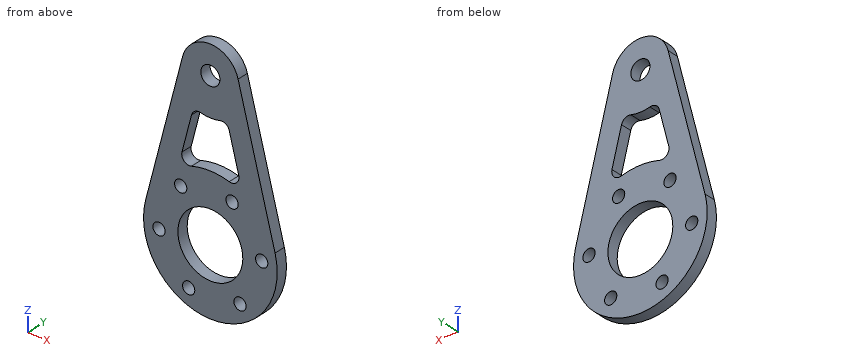
```python
from build123d import *

# Parameters (mm, degrees)
SKETCH_1_R               = 17.5
SKETCH_1_R_2             = 7.5
SKETCH_1_R_3             = 2.5
EXTRUDE_1_DEPTH          = 3
SKETCH_2_R               = 1.6
SKETCH_2_R_2             = 8.5
CUT_EXTRUDE_1_DEPTH      = 4
PATTERN_CIRCULAR_1_COUNT = 2
CUT_EXTRUDE_2_DEPTH      = 4
FILLET_1_R               = 2


with BuildPart() as part:
    # 草图1 → 凸台-拉伸1 (new body)
    # profile 1 of 3: a face of its own
    with BuildSketch(Plane(origin=(0, 0, 0), x_dir=(1, 0, 0), z_dir=(0, 1, 0))):
        Circle(SKETCH_1_R)
    # profile 2 of 3: a face of its own
    with BuildSketch(Plane(origin=(0, 0, 0), x_dir=(1, 0, 0), z_dir=(0, 1, 0))):
        with BuildLine():
            Line((-16.94430214, -4.375), (-7.261843774, -41.875))
            ThreePointArc((-7.261843774, -41.875), (-0.945032194, -32.559777278), (7.5, -40))
            ThreePointArc((7.5, -40), (7.440222722, -40.945032194), (7.261843774, -41.875))
            Line((7.261843774, -41.875), (16.94430214, -4.375))
            ThreePointArc((16.94430214, -4.375), (0, -17.5), (-16.94430214, -4.375))
        make_face()
    # profile 3 of 3: a face of its own
    with BuildSketch(Plane(origin=(0, 0, 0), x_dir=(1, 0, 0), z_dir=(0, 1, 0))):
        with Locations((0, -40)):
            Circle(SKETCH_1_R_2)
        with Locations(Location((0, -40, 0), (0, 0, 270))):
            Circle(SKETCH_1_R_3, mode=Mode.SUBTRACT)
    extrude(amount=EXTRUDE_1_DEPTH)

    # 草图2 → 切除-拉伸1 (cut)
    with BuildSketch(Plane.XZ):
        with Locations(Location((13.446267609, 1.203281922, 0), (0, 0, 270))):
            Circle(SKETCH_2_R)
        with Locations(Location((-5.681061093, -12.246450296, 0), (0, 0, 270))):
            Circle(SKETCH_2_R)
        with Locations(Location((-7.765206517, 11.043168375, 0), (0, 0, 270))):
            Circle(SKETCH_2_R)
        with Locations(Location((0, 0, 0), (0, 0, 270))):
            Circle(SKETCH_2_R_2)
    cut_extrude_1 = extrude(amount=-CUT_EXTRUDE_1_DEPTH, mode=Mode.SUBTRACT)

    # 阵列(圆周)1: 切除-拉伸1 ×2 about axis
    pattern_circular_1_axis = Axis((0, 0, 0), (0, 1, 0))
    for i in range(1, PATTERN_CIRCULAR_1_COUNT):
        add(cut_extrude_1.rotate(pattern_circular_1_axis, i * 360 / PATTERN_CIRCULAR_1_COUNT), mode=Mode.SUBTRACT)

    # 草图3 → 切除-拉伸2 (cut)
    with BuildSketch(Plane.XZ):
        with BuildLine():
            ThreePointArc((-8.434515238, 15.33326295), (0, 17.5), (8.434515238, 15.33326295))
            Line((8.434515238, 15.33326295), (4.385981416, 31.013167019))
            ThreePointArc((4.385981416, 31.013167019), (0, 30), (-4.385981416, 31.013167019))
            Line((-4.385981416, 31.013167019), (-8.434515238, 15.33326295))
        make_face()
    extrude(amount=-CUT_EXTRUDE_2_DEPTH, mode=Mode.SUBTRACT)

    # 圆角1
    fillet_1_edges = [part.edges().sort_by_distance(p)[0] for p in [
        (-4.385981416, 1.5, 31.013167019),
        (4.385981416, 1.5, 31.013167019),
        (8.434515238, 1.5, 15.33326295),
        (-8.434515238, 1.5, 15.33326295),
    ]]
    fillet(fillet_1_edges, radius=FILLET_1_R)


solid = part.part
```
Here's how the part is built. I have some questions about the finished solid (model axes, mm). Give positions to 0.01 mm unless a question says otherwise; leave off trailing zeros. Write each loop counter-clockwise with the first axis right and the second up, starting at its lowest first coordinate (ties: lowest second). Pieces come first, ordered by that corner, then holes.
(1) If I drill on L1, parallel to Z at x = 3.5, y = 0.7; L2, parallel to Z at x = -0.5, y = 2.6; L3, parallel to Z at x = -1, y = 2.8, over which ranges is the centre line in solid material (lowest first)?
Output values:
L1: z = -17.15 to -7.75, 7.75 to 17.15, 30.32 to 46.63
L2: z = -17.49 to -8.49, 8.49 to 17.49, 30.01 to 37.55, 42.45 to 47.48
L3: z = -17.47 to -8.44, 8.44 to 17.47, 30.05 to 37.71, 42.29 to 47.43
(2) Imagine slicing it at A-A, the plane x = 0. Write out the boundary of the cut face in (y, z), and give its area (3 significant figures).
Output values:
outline: (0, -17.5) - (3, -17.5) - (3, -8.5) - (0, -8.5) - close; (0, 8.5) - (3, 8.5) - (3, 17.5) - (0, 17.5) - close; (0, 30) - (3, 30) - (3, 37.5) - (0, 37.5) - close; (0, 42.5) - (3, 42.5) - (3, 47.5) - (0, 47.5) - close
area: 91.5 mm2
(3) Imagine slicing it at C-C, the plane z = 40. Write out the boundary of the cut face in (x, y), and give its area (3 significant figures).
Output values:
outline: (-7.75, 0) - (-2.5, 0) - (-2.5, 3) - (-7.75, 3) - close; (2.5, 0) - (7.75, 0) - (7.75, 3) - (2.5, 3) - close
area: 31.5 mm2
(4) Imagine slicing it at D-D, the plane x = 12.5. Write out the boundary of the cut face in (y, z), and give its area (3 significant figures).
Output values:
outline: (0, -12.25) - (3, -12.25) - (3, -0.09) - (0, -0.09) - close; (0, 2.49) - (3, 2.49) - (3, 21.59) - (0, 21.59) - close
area: 93.8 mm2
(5) Imagine slicing it at B-B, the plane y = 0.65. Count the separate pieces of the cut face and the enclosed holes in it, and give its area (3 significant figures).
Output values:
separate pieces: 1
enclosed holes: 9
area: 1,140 mm2
